Verification items for the finished model (mm, model axes). A direction names the side the tool comes from. Give positions to 0.01 mm unless a question says otherwise; leave off trailing zeros. Order: outer loops, then holes, each group sorted by start corner. A loop starts at its lowest first (then second) coordinate and runs counter-clockwise, first axis right, second up.
Autodesk Inventor part; units mm, degrees
ref_plane "YZ Plane" through (0, 0, 0) normal (1, 0, 0) x (0, 1, 0)
ref_plane "XZ Plane" through (0, 0, 0) normal (0, 1, 0) x (-1, 0, 0)
ref_plane "XY Plane" through (0, 0, 0) normal (0, 0, 1) x (1, 0, 0)
sketch "Sketch2" plane through (0, 0, 0) normal (1, 0, 0) x (0, 1, 0)
  line L0 (0, 0) -> (32, 0)
  line L1 (0, 0) -> (-8, -23.4)
  line L2 (-8, -23.4) -> (16, -23.4)
  line L3 (16, -23.4) -> (32, 0)
  dimension "d4" = 32
  dimension "d32" = 24
  dimension "d34" = 8
  dimension "d35" = 23.4
extrude "Extrusion1" add sketch "Sketch2" along normal blind 8
sketch "Sketch7" plane through (0, -8, -23.4) normal (0, 0, -1) x (-1, 0, 0)
  line L0 (0, 24) -> (-8, 24)
  line L1 (-8, 24) -> (0, 24)
  line L2 (0, 24) -> (0, 16.3)
  line L3 (0, 16.3) -> (-8, 16.3)
  line L4 (-8, 16.3) -> (-8, 24)
  line L5 (0, 0) -> (-8, 0)
  line L6 (-8, 0) -> (0, 0)
  line L7 (0, 0) -> (0, 7.7)
  line L8 (0, 7.7) -> (-8, 7.7)
  line L9 (-8, 7.7) -> (-8, 0)
  point P0 (0, 8)
  dimension "d36" = 8
  dimension "d37" = 7.7
  dimension "d38" = 8
  dimension "d39" = 7.7
extrude "Extrusion6" add sketch "Sketch7" along normal blind 8.3
sketch "Sketch8" plane through (0, 0, 0) normal (0, 0, 1) x (1, 0, 0)
  line L0 (0, 32) -> (8, 32)
  line L1 (8, 32) -> (0, 32)
  line L2 (0, 32) -> (0, 24.3)
  line L3 (0, 24.3) -> (8, 24.3)
  line L4 (8, 24.3) -> (8, 32)
  line L5 (8, 0) -> (0, 0)
  line L6 (0, 0) -> (0, 7.7)
  line L7 (0, 7.7) -> (8, 7.7)
  line L8 (8, 7.7) -> (8, 0)
  dimension "d42" = 8
  dimension "d43" = 7.7
  dimension "d44" = 8
  dimension "d45" = 7.7
extrude "Extrusion7" add sketch "Sketch8" along normal blind 8.3
sketch "Sketch9" plane through (0, 24.3, 0) normal (0, -1, 0) x (1, 0, 0)
  circle A0 centre (4, 4.3) radius 2.3
  line L0 (0, 0) -> (0, 8.3)
  line L1 (0, 8.3) -> (8, 8.3)
  dimension "d48" = 4.6
  dimension "d49" = 4
  dimension "d50" = 4
extrude "Extrusion8" add sketch "Sketch9" along normal up to surface (16.6 mm away)
sketch "Sketch10" plane through (0, 16, -23.4) normal (0, 1, 0) x (1, 0, 0)
  circle A0 centre (4, 4.3) radius 2.5
  line L0 (8, 0) -> (8, 8.3)
  line L1 (0, 8.3) -> (8, 8.3)
  point P0 (0, -23.4)
  dimension "d53" = 5
  dimension "d54" = 4
  dimension "d55" = 4
extrude "Extrusion9" cut sketch "Sketch10" against normal up to surface (24 mm away)
fillet "Fillet2" radius 4 8 edges at (0, 12.15, -31.7) (8, 12.15, -31.7) (8, -4.15, -31.7) (0, -4.15, -31.7) (0, 28.15, 8.3) (0, 3.85, 8.3) (8, 28.15, 8.3) (8, 3.85, 8.3)
properties part number "Crank1"
(1) Set-up check for faces 5 (the flat face through (4, 4, -23.4)), 6 (the cylindrical face through (1.203, 28.096, 7.159)), 7 (the flat face through (4, 16, 0)), 8 (the flat face through (6, 24.3, 2)): record each of +Z, -Z, +X, -X, +Y, -Y from which the full face is reachable in a straight line by a thin tool's end or side.
Solved:
face 5: -Z, +X, -X
face 6: +Z, -X, +Y, -Y
face 7: +X, -X
face 8: none
(2) Section check C-C, the plane x = 3.25. Enter the section's corners in (y, z), then the cut area to 3 significant figures.
Solved:
outline: (-8, -31.63) - (-0.3, -31.63) - (-0.3, -30.08) - (-8, -30.08) - close; (-8, -25.32) - (-0.3, -25.32) - (-0.3, -23.4) - (8.3, -23.4) - (8.3, -25.32) - (16, -25.32) - (16, -23.4) - (32, 0) - (32, 8.23) - (24.3, 8.23) - (24.3, 6.47) - (7.7, 6.47) - (7.7, 8.23) - (0, 8.23) - (0, 0) - (-8, -23.4) - close; (8.3, -31.63) - (16, -31.63) - (16, -30.08) - (8.3, -30.08) - close; hole (7.7, 0) - (24.3, 0) - (24.3, 2.13) - (7.7, 2.13) - close
area: 907 mm2
(3) Section check D-D, the plane y = 19. Enter the section's corners in (x, z), then the cut area to 3 significant figures.
Solved:
outline: (0, -19.01) - (8, -19.01) - (8, 0) - (0, 0) - close; circle Ø4.6 at (4, 4.3)
area: 169 mm2
(4) Go/stop test with flat-tipped pins: pin 1 (4 mm diameter, centred on x = 3.5, y = 26.5, fed in from +Z); pin 2 (1.5 mm diameter, centred on x = 6.5, z = -5.5, fed in from +Y); pin 3 (2.5 mm diameter, centred on x = 4, y = 14, fed in from +Z); pin 4 (4.5 mm diameter, centred on x = 4, z = -27.7, fed in from -Y). Record where each tip stops, or that it passes through.
Solved:
pin 1: stops at z = 8.3
pin 2: stops at y = 28.75
pin 3: stops at z = 6.6
pin 4: passes through
(5) Section check A-A, the plane y = 14.5. Give the number of separate pieces and of enclosed holes in the cut face, then the cut area to 3 significant figures.
Solved:
separate pieces: 2
enclosed holes: 1
area: 244 mm2
(6) Release check for a two-part mould opening along Y. For faces 1 (the flat face through (6, 7.7, 2)), 2 (the flat face through (5.7, -0.3, -25.6)), 3 (the flat face through (8, 12, -11)), 4 (the flat face through (5.7, -8, -25.6)) record: pulls with the +Y half, pulls with the -Y half, needs draft (parallel to the pull), parting line crosses it, or undercut.
Solved:
face 1: undercut
face 2: undercut
face 3: needs draft
face 4: pulls with the -Y half
(7) Scan lines: line 1 (Z direction, x = 4, y = 13); line 2 (X direction, y = -5.25, z = -27.7); line 3 (Y direction, x = 7.75, z = -25.5). Record each from-to range of solid material in increasing order.
Solved:
line 1: z = -31.7 to -30.2, -25.2 to 0, 2 to 6.6
line 2: x = 0 to 1.5, 6.5 to 8
line 3: y = -8 to -0.3, 8.3 to 16
(8) Section check B-B, the plane z = 0.5. Enter the section's corners in (x, y).
Solved:
outline: (0, 0) - (8, 0) - (8, 7.7) - (0, 7.7) - close; (0, 24.3) - (8, 24.3) - (8, 32) - (0, 32) - close
